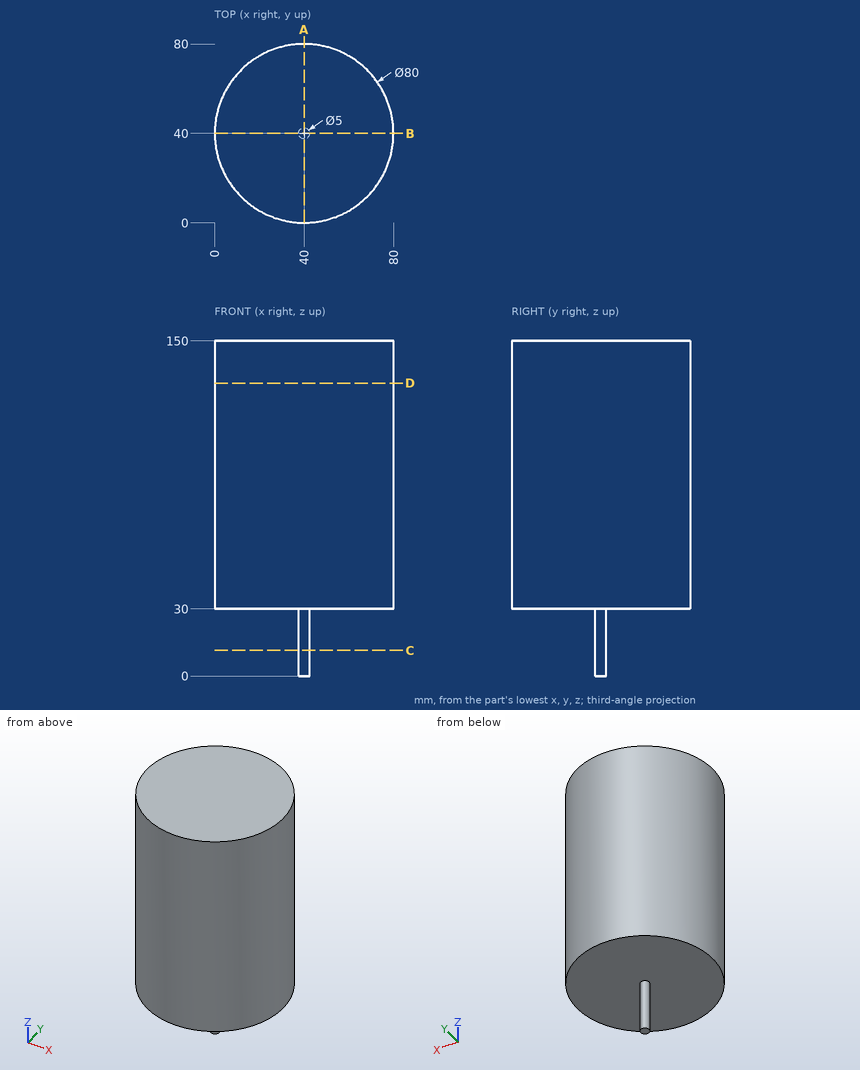
Part print with two shaded views. Sizes in mm from the minimum x, y, z corner. Round coordinates to 2 decimals unless told otherwise and drop trailing zeros. Order: outer loops, then holes, each group sorted by start corner. A loop starts at its lowest first (then second) coordinate and runs counter-clockwise, first axis right, second up. Notation, with made-up numbers: M 50.25,88.5 L 100.25,88.5 A20 ccw 100.25,121.5 Z; hole C 50.5,-35.75 d11. An arc over 180 degrees is marked long. Answer in a Markdown table with one row per item. Add a question column.
Q1. Cut at D-D on z = 131. Give the cut face in (x, y).
Q2. Pin check, flat tips, straight feed: pin 1 (2 mm diameter, centred on x = 44.5, z = 66, fed in from +Y); pin 2 (1 mm diameter, centred on x = 8.5, y = 13, fed in from -Z); pin 3 (2 mm diameter, centred on x = 22.5, z = 54.5, fed in from +Y); pin 4 (2 mm diameter, centred on x = 10, z = 133, fed in from -Y). Stop position of each tip, or through.
Q3. Cut at C-C on z = 11.5. Give the cut face in (x, y), and give its area (3 significant figures).
Q4. Cut at A-A on x = 40. Give the cut face in (y, z).
Q5. Wall check: L1, parallel to Z at x = 66, y = 53.5; L2, parallel to Y at x = 32.5, z = 47; L3, parallel to X at y = 60.5, z = 42. Give the ranges that are in metal, low to high. Write a range as from..to.
Established:
| question | item | result |
|---|---|---|
| 1 | outline | C 40,40 d80 |
| 2 | pin 1 | stops at y = 79.85 |
| 2 | pin 2 | passes through |
| 2 | pin 3 | stops at y = 76.44 |
| 2 | pin 4 | stops at y = 12.45 |
| 3 | outline | C 40,40 d5 |
| 3 | area | 19.6 mm2 |
| 4 | outline | M 0,30 L 37.5,30 L 37.5,0 L 42.5,0 L 42.5,30 L 80,30 L 80,150 L 0,150 Z |
| 5 | L1 | z = 30..150 |
| 5 | L2 | y = 0.71..79.29 |
| 5 | L3 | x = 5.65..74.35 |
